Job drawing, mm, ordinate dimensions from the low corner. One solid piece. Round coordinates to 2 decimals unless told otherwise and drop trailing zeros. Loops run counter-clockwise (first coordinate to the right, second up) from the corner with the lowest first, then second, coordinate; pieces in that order, holes last.
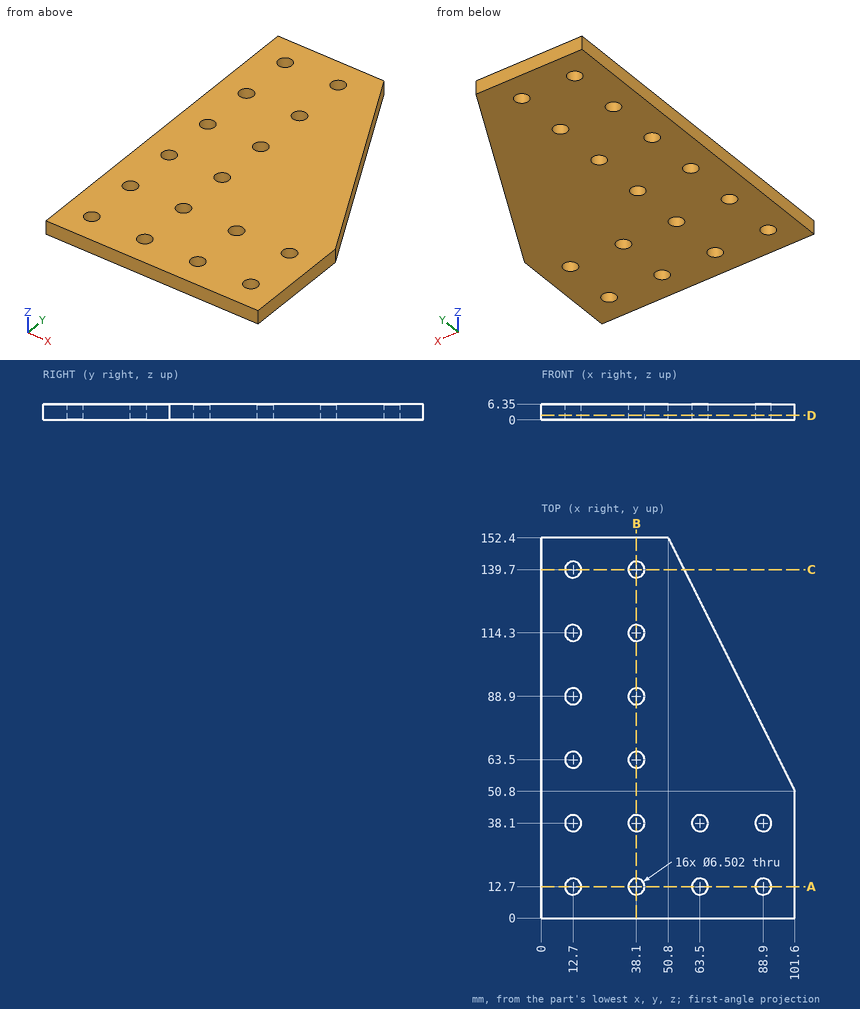
Item 1: Cut at C-C, the plane y = 139.7. Give the cut face in (x, z), plus the area to 3 significant figures.
Answers follow:
outline: (0, 0) - (9.45, 0) - (9.45, 6.35) - (0, 6.35) - close; (15.95, 0) - (34.85, 0) - (34.85, 6.35) - (15.95, 6.35) - close; (41.35, 0) - (57.15, 0) - (57.15, 6.35) - (41.35, 6.35) - close
area: 280 mm2
Item 2: Flat gauge pins, fed straight in: P1, Ø8.5, axis at x = 12.7, y = 114.3, coming from the -Z side; P2, Ø4, axis at x = 38.1, y = 139.7, coming from the -Z side. Where does each tip first touch, or does it go through?
Answers follow:
P1: stops at z = 0
P2: passes through
Item 3: Cut at D-D, the plane z = 1.75. State how many separate pieces and enclosed holes the cut face has, plus the area to 3 significant figures.
Answers follow:
separate pieces: 1
enclosed holes: 16
area: 12,400 mm2
Item 4: Cut at A-A, the plane y = 12.7. Give the cut face in (x, z).
Answers follow:
outline: (0, 0) - (9.45, 0) - (9.45, 6.35) - (0, 6.35) - close; (15.95, 0) - (34.85, 0) - (34.85, 6.35) - (15.95, 6.35) - close; (41.35, 0) - (60.25, 0) - (60.25, 6.35) - (41.35, 6.35) - close; (66.75, 0) - (85.65, 0) - (85.65, 6.35) - (66.75, 6.35) - close; (92.15, 0) - (101.6, 0) - (101.6, 6.35) - (92.15, 6.35) - close
Item 5: Probe line 1 (Y direction, x = 65.5, z = 5.5) (1 decimal); line 2 (Y direction, x = 91, z = 4.5) (1 decimal); line 3 (X direction, y = 141, z = 4). List the from-to ranges inside material, lowest first.
Answers follow:
line 1: y = 0 to 10.1, 15.3 to 35.5, 40.7 to 123
line 2: y = 0 to 10.2, 15.2 to 35.6, 40.6 to 72
line 3: x = 0 to 9.72, 15.68 to 35.12, 41.08 to 56.5
Item 6: Cut at B-B, the plane x = 38.1. Give the cut face in (y, z), plus the area to 3 significant figures.
Answers follow:
outline: (0, 0) - (9.45, 0) - (9.45, 6.35) - (0, 6.35) - close; (15.95, 0) - (34.85, 0) - (34.85, 6.35) - (15.95, 6.35) - close; (41.35, 0) - (60.25, 0) - (60.25, 6.35) - (41.35, 6.35) - close; (66.75, 0) - (85.65, 0) - (85.65, 6.35) - (66.75, 6.35) - close; (92.15, 0) - (111.05, 0) - (111.05, 6.35) - (92.15, 6.35) - close; (117.55, 0) - (136.45, 0) - (136.45, 6.35) - (117.55, 6.35) - close; (142.95, 0) - (152.4, 0) - (152.4, 6.35) - (142.95, 6.35) - close
area: 720 mm2
